Autodesk Inventor part; units mm, degrees
ref_plane "Work Plane1" through (0, 14, 323.5) normal (0, 1, 0) x (-1, 0, 0)
ref_plane "YZ Plane" through (0, 0, 0) normal (1, 0, 0) x (0, 1, 0)
ref_plane "XY Plane" through (0, 0, 0) normal (0, 0, 1) x (1, 0, 0)
sketch "Sketch1" plane through (0, 0, 0) normal (0, 0, 1) x (1, 0, 0)
  line L0 (-9.2376, -16) -> (-18.4752, 0)
  line L1 (-18.4752, 0) -> (-9.2376, 16)
  line L2 (-9.2376, 16) -> (9.2376, 16)
  line L3 (9.2376, 16) -> (18.4752, 0)
  line L4 (18.4752, 0) -> (9.2376, -16)
  line L5 (9.2376, -16) -> (-9.2376, -16)
  point P0 (0, 0)
  point P1 (0, 0)
  dimension "d0" = 32
extrude "Extrusion1" add sketch "Sketch1" along normal mid plane 334
sketch "Sketch3" plane through (0, 0, 0) normal (0, 1, 0) x (-1, 0, 0)
  line L0 (0, -227) -> (0, 0)
  line L1 (0, 0) -> (0, 420)
  line L2 (0, 420) -> (-14, 420)
  line L3 (-14, 420) -> (-14, 227)
  line L4 (-14, 227) -> (-15, 227)
  line L5 (-15, 227) -> (-15, 0)
  line L6 (-15, 0) -> (-15, -227)
  line L7 (-15, -227) -> (0, -227)
  line L8 (-15, -223) -> (-14, -223)
  line L9 (-14, -223) -> (-14, -221)
  line L10 (-14, -221) -> (-15, -221)
  line L11 (-15, -221) -> (-15, -223)
  line L12 (-14, 416) -> (-13, 416)
  line L13 (-13, 416) -> (-13, 414)
  line L14 (-13, 414) -> (-14, 414)
  line L15 (-14, 414) -> (-14, 416)
  line L16 (-15, 223) -> (-14, 223)
  line L17 (-14, 223) -> (-14, 221)
  line L18 (-14, 221) -> (-15, 221)
  line L19 (-15, 221) -> (-15, 223)
  point P0 (-15, 221)
  dimension "d8" = 30
  dimension "d9" = 227
  dimension "d10" = 420
  dimension "d12" = 28
  dimension "d14" = 4
  dimension "d15" = 2
  dimension "d16" = 26
  dimension "d17" = 2
  dimension "d18" = 4
  dimension "d19" = 28
  dimension "d20" = 227
  dimension "d21" = 2
  dimension "d22" = 4
  dimension "d23" = 28
revolve "Revolution1" add sketch "Sketch3" angle 360 about axis through (0, 0, -227) along (0, 0, 1) contours L7 L6 L8 L9 L10 L5 L18 L17 L16 L4 L3 L14 L13 L12 L2 L1 L0 | L12 L13 L14 L3
ref_plane "Work Plane1" through (0, 14, 323.5) normal (0, 1, 0) x (-1, 0, 0)
sketch "Sketch4" plane through (0, 14, 323.5) normal (0, 1, 0) x (-1, 0, 0)
  line L0 (14, -96.5) -> (-14, -96.5) construction
  line L1 (14, 96.5) -> (-14, 96.5) construction
  line L2 (0, 86.5) -> (0, -33.5) construction
  line L3 (-4, 86.5) -> (-4, -33.5)
  line L4 (4, -33.5) -> (4, 86.5)
  arc A0 (4, 86.5) -> (-4, 86.5) centre (0, 86.5) ccw
  arc A1 (-4, -33.5) -> (4, -33.5) centre (0, -33.5) ccw
  point P0 (0, -323.5)
  point P1 (0, 26.5)
  point P2 (0, 96.5)
  dimension "d24" = 8
  dimension "d25" = 10
  dimension "d26" = 120
extrude "Extrusion3" cut sketch "Sketch4" against normal blind 4
equation "\"d23\" = d19"
properties part number "NVPH-201 shredder shaft"
Here's how the part is built. I have some questions about the finished solid (model axes, mm). A direction names the side the tool comes from. Coordinates: 2 decimals unless noted, no trailing zeros. Write each loop counter-clockwise with the first axis right and the second up, starting at its lowest first coordinate (ties: lowest second). Pieces come first, ordered by that corner, then holes. Notation, with made-up numbers: (-24.5, 35.25) - (4.5, 35.25) arc R34 cw to (4.5, 74.25) - close; hole circle Ø8 at (42.25, -18). An arc over 180 degrees is marked (long way). One line per item, written item: value.
1) On a 3-axis mill with a long thin cutter (end or side, diameter ignored), from which of +Z, -Z, +X, -X, +Y, -Y can I reach the whole of each face in a straight line? I mean faces 1 (the cylindrical face through (12.932, -5.362, -221.986)), 2 (the cylindrical face through (-14.985, -0.66, -194.378)), 3 (the flat face through (13.92, -7.89, -2.34)), 4 (the flat face through (0, 0, 420)), 5 (the cylindrical face through (7.526, -11.805, 322.149)). Say none if no direction works.
Model answer:
face 1: none
face 2: -Z
face 3: +Z, -Z, +X, -Y
face 4: +Z, +X, -X, +Y, -Y
face 5: +Z
2) I need wall thicknesses on line 1 along Z through (x, y) = (9, -11); line 2 along X through (y, z) = (-10.5, 357); line 3 along Y through (x, z) = (-1, 327). Which ranges of each line are inside material? Lowest first, please.
Model answer:
line 1: z = -227 to -223, -221 to 221, 223 to 227
line 2: x = -9.26 to 9.26
line 3: y = -13.96 to 10
3) I'm going to push flat-ended pins straight in: P1, Ø9, axis at x = 2, z = 330.5, coming from the +Y side; P2, Ø5, axis at y = 12.5, z = 180, coming from the -X side; P3, Ø4, axis at y = 6, z = 9, coming from the +X side. Where does each tip first touch, or does it pass through?
Model answer:
P1: stops at y = 13.42
P2: stops at x = -11.18
P3: stops at x = 16.17
4) Suppose I cut it at A-A on z = -138.5. Write out the boundary of the cut face in (x, y).
Model answer:
outline: (-18.48, 0) - (-9.24, -16) - (9.24, -16) - (18.48, 0) - (9.24, 16) - (-9.24, 16) - close
5) We'd pull the mould along Z, two halves only. Please class faces 6 (the flat face through (0, 0, -227)), 7 (the cylindrical face through (12.932, 5.362, 221.986)), 8 (the flat face through (0, -16, -2)): pulls with the +Z half, pulls with the -Z half, needs draft (parallel to the pull), parting line crosses it, or undercut.
Model answer:
face 6: pulls with the -Z half
face 7: undercut
face 8: needs draft
6) Suppose I cut it at C-C on z = 349.5. Write out the boundary of the cut face in (x, y), and give its area (3 significant figures).
Model answer:
outline: (-4, 10) - (-4, 13.42) arc R14 ccw (long way) to (4, 13.42) - (4, 10) - close
area: 585 mm²
